CAD build for the part. Positions are in the model's coordinates, mm. A direction names the side the tool comes from. Round coordinates to 2 decimals unless told otherwise and drop trailing zeros. Loops run counter-clockwise (first coordinate to the right, second up) from the corner with the lowest first, then second, coordinate; pieces in that order, holes last. Notation, with made-up numbers: (-36, 13.25) - (13, 13.25) arc R18 ccw to (13, 22.25) - close; hole circle Ø4 at (32.5, 9.25). An arc over 180 degrees is marked (long way). One line per question, with ' | ' between items.
```python
from build123d import *

# Parameters (mm, degrees)
F1_DEPTH      = 12.7
F1_DEPTH_BACK = 12.7
F0_R          = 1.778
F2_DEPTH      = 2.286
F2_DEPTH_BACK = 2.286
F4_R          = 1.778
F5_DEPTH      = 3.81
F7_R          = 1.778
F8_DEPTH      = 3.81


with BuildPart() as f1:
    # F0 (on Right) → F1 (new body, two sides)
    with BuildSketch(Plane.YZ) as f1_sk:
        Polygon((20.2659536765, 17.9712367281), (-30.5340463235, 17.9712367281), (-30.5340463235, 15.8122367281), (13.4079536765, 15.8122367281), (20.2659536765, 15.8122367281), align=None)
    extrude(amount=F1_DEPTH)
    extrude(f1_sk.sketch, amount=-F1_DEPTH_BACK)

    # F0 (on Right) → F2 (join, two sides)
    with BuildSketch(Plane.YZ) as f2_sk:
        with BuildLine():
            Line((20.2659536765, 11.6212367281), (20.2659536765, 15.8122367281))
            Line((20.2659536765, 15.8122367281), (13.4079536765, 15.8122367281))
            Line((13.4079536765, 15.8122367281), (13.4079536765, 11.6212367281))
            ThreePointArc((13.4079536765, 11.6212367281), (16.8369536765, 15.0502367281), (20.2659536765, 11.6212367281))
        make_face()
        with BuildLine():
            ThreePointArc((13.4079536765, 11.6212367281), (16.8369536765, 8.1922367281), (20.2659536765, 11.6212367281))
            ThreePointArc((20.2659536765, 11.6212367281), (16.8369536765, 15.0502367281), (13.4079536765, 11.6212367281))
        make_face()
        with Locations((16.8369536765, 11.6212367281)):
            Circle(F0_R, mode=Mode.SUBTRACT)
    extrude(amount=F2_DEPTH)
    extrude(f2_sk.sketch, amount=-F2_DEPTH_BACK)

    # F4 (on offset) → F5 (join)
    with BuildSketch(Plane.YZ.offset(9.525)):
        with BuildLine():
            Line((20.2659536765, 15.8122367281), (13.4079536765, 15.8122367281))
            Line((13.4079536765, 15.8122367281), (13.4079536765, 11.6212367281))
            ThreePointArc((13.4079536765, 11.6212367281), (16.8369536765, 8.1922367281), (20.2659536765, 11.6212367281))
            Line((20.2659536765, 11.6212367281), (20.2659536765, 15.8122367281))
        make_face()
        with Locations((16.8369536765, 11.6212367281)):
            Circle(F4_R, mode=Mode.SUBTRACT)
    extrude(amount=-F5_DEPTH)

    # F7 (on offset) → F8 (join)
    with BuildSketch(Plane(origin=(-9.525, 0, 0), x_dir=(0, -1, 0), z_dir=(-1, 0, 0))):
        with BuildLine():
            Line((-13.4079536765, 11.6212367281), (-13.4079536765, 15.8122367281))
            Line((-13.4079536765, 15.8122367281), (-20.2659536765, 15.8122367281))
            Line((-20.2659536765, 15.8122367281), (-20.2659536765, 11.6212367281))
            ThreePointArc((-20.2659536765, 11.6212367281), (-16.8369536765, 8.1922367281), (-13.4079536765, 11.6212367281))
        make_face()
        with Locations((-16.8369536765, 11.6212367281)):
            Circle(F7_R, mode=Mode.SUBTRACT)
    extrude(amount=-F8_DEPTH)


solid = f1.part
```
(1) Cut at A-A, the plane x = -6.25. Write the cut outline in (y, z), then the cut area to 3 significant figures.
Results found:
outline: (-30.53, 15.81) - (13.41, 15.81) - (13.41, 11.62) arc R3.43 ccw to (20.27, 11.62) - (20.27, 17.97) - (-30.53, 17.97) - close; hole circle Ø3.56 at (16.84, 11.62) | area: 147 mm²
(2) Tool access for faces 4 (the face through (-9.525, 17, 14)), 5 (the face through (7.647, 15.526, 12.823)), 6 (the face through (-8, 13.408, 14)), 7 (the face through (2.286, 17, 14)), 8 (the face through (0, -5, 17.971)): list every direction of +Z, -Z, +X, -X, +Y, -Y with a clear straight run to the whole face (end or side of a thin tool).
Results found:
face 4: -Z, -X, +Y, -Y | face 5: +X, -X | face 6: -Z, +X, -X, -Y | face 7: -Z, +Y, -Y | face 8: +Z, +X, -X, +Y, -Y
(3) Drop flat-ended pins along their axis: P1, Ø5.5, axis at y = 16.84, z = 11.62, coming from the +X side (3 decimals); P2, Ø3, axis at x = -6.5, z = 14, coming from the -Y side; P3, Ø3.5, axis at y = 18.5, z = 10.5, coming from the -X side (3 decimals); P4, Ø2, axis at y = -25.5, z = 15.5, coming from the -X side. Give the stop position or say it passes through.
Results found:
P1: stops at x = 9.525 | P2: stops at y = 13.41 | P3: stops at x = -9.525 | P4: stops at x = -12.7
(4) Probe L1, parallel to Z at x = 8.5, y = 17; L2, parallel to Z at x = -0.5, y = -14; L3, parallel to Y at x = 1, z = 14.5. List the from-to ranges inside material, lowest first.
Results found:
L1: z = 8.2 to 9.85, 13.39 to 17.97 | L2: z = 15.81 to 17.97 | L3: y = 13.41 to 20.27
(5) Cut at D-D, the plane y = 12.5. Write the cut outline in (x, z), then the cut area to 3 significant figures.
Results found:
outline: (-12.7, 15.81) - (12.7, 15.81) - (12.7, 17.97) - (-12.7, 17.97) - close | area: 54.8 mm²
(6) Two-plate mould, pull along X, no slides. Class faces 1 (the face through (9.525, 17, 14)), 2 (the face through (-2.286, 17, 14)), 3 (the face through (0.032, 16.762, 8.193)): released by +X, released by -X, zero draft, split by the parting line, or undercut.
Results found:
face 1: released by +X | face 2: undercut | face 3: zero draft
(7) Cut at B-B, the plane z = 9. Write the cut outline in (x, y) (3 decimals).
Results found:
outline: (-9.525, 14.626) - (-5.715, 14.626) - (-5.715, 19.048) - (-9.525, 19.048) - close; (-2.286, 14.626) - (2.286, 14.626) - (2.286, 19.048) - (-2.286, 19.048) - close; (5.715, 14.626) - (9.525, 14.626) - (9.525, 19.048) - (5.715, 19.048) - close
(8) Cut at C-C, the plane z = 12.75. Write the cut outline in (x, y) (3 decimals).
Results found:
outline: (-9.525, 13.408) - (-5.715, 13.408) - (-5.715, 15.463) - (-9.525, 15.463) - close; (-9.525, 18.211) - (-5.715, 18.211) - (-5.715, 20.266) - (-9.525, 20.266) - close; (-2.286, 13.408) - (2.286, 13.408) - (2.286, 15.463) - (-2.286, 15.463) - close; (-2.286, 18.211) - (2.286, 18.211) - (2.286, 20.266) - (-2.286, 20.266) - close; (5.715, 13.408) - (9.525, 13.408) - (9.525, 15.463) - (5.715, 15.463) - close; (5.715, 18.211) - (9.525, 18.211) - (9.525, 20.266) - (5.715, 20.266) - close
